Autodesk Inventor part; units mm, degrees
ref_plane "YZ Plane" through (0, 0, 0) normal (1, 0, 0) x (0, 1, 0)
ref_plane "XZ Plane" through (0, 0, 0) normal (0, 1, 0) x (-1, 0, 0)
ref_plane "XY Plane" through (0, 0, 0) normal (0, 0, 1) x (1, 0, 0)
sketch "Boceto1" plane through (0, 0, 0) normal (0, 0, 1) x (1, 0, 0)
  arc A0 (-116.1173, 21.3488) -> (-117.6673, 19.7988) centre (-116.1173, 19.7988) ccw
  arc A1 (-117.6673, 19.7988) -> (-116.1173, 18.2488) centre (-116.1173, 19.7988) ccw
  arc A2 (-116.1173, 18.2488) -> (-114.5673, 19.7988) centre (-116.1173, 19.7988) ccw
  arc A3 (-114.5673, 19.7988) -> (-116.1173, 21.3488) centre (-116.1173, 19.7988) ccw
  arc A4 (-67.1173, 21.3488) -> (-68.6673, 19.7988) centre (-67.1173, 19.7988) ccw
  arc A5 (-68.6673, 19.7988) -> (-67.1173, 18.2488) centre (-67.1173, 19.7988) ccw
  arc A6 (-67.1173, 18.2488) -> (-65.5673, 19.7988) centre (-67.1173, 19.7988) ccw
  arc A7 (-65.5673, 19.7988) -> (-67.1173, 21.3488) centre (-67.1173, 19.7988) ccw
  arc A8 (-18.1173, 21.3488) -> (-19.6673, 19.7988) centre (-18.1173, 19.7988) ccw
  arc A9 (-19.6673, 19.7988) -> (-18.1173, 18.2488) centre (-18.1173, 19.7988) ccw
  arc A10 (-18.1173, 18.2488) -> (-16.5673, 19.7988) centre (-18.1173, 19.7988) ccw
  arc A11 (-16.5673, 19.7988) -> (-18.1173, 21.3488) centre (-18.1173, 19.7988) ccw
  arc A12 (-18.1173, -7.6512) -> (-19.6673, -9.2012) centre (-18.1173, -9.2012) ccw
  arc A13 (-19.6673, -9.2012) -> (-18.1173, -10.7512) centre (-18.1173, -9.2012) ccw
  arc A14 (-18.1173, -10.7512) -> (-16.5673, -9.2012) centre (-18.1173, -9.2012) ccw
  arc A15 (-16.5673, -9.2012) -> (-18.1173, -7.6512) centre (-18.1173, -9.2012) ccw
  arc A16 (-116.1173, -7.6512) -> (-117.6673, -9.2012) centre (-116.1173, -9.2012) ccw
  arc A17 (-117.6673, -9.2012) -> (-116.1173, -10.7512) centre (-116.1173, -9.2012) ccw
  arc A18 (-116.1173, -10.7512) -> (-114.5673, -9.2012) centre (-116.1173, -9.2012) ccw
  arc A19 (-114.5673, -9.2012) -> (-116.1173, -7.6512) centre (-116.1173, -9.2012) ccw
  arc A20 (-116.1173, -36.6512) -> (-117.6673, -38.2012) centre (-116.1173, -38.2012) ccw
  arc A21 (-117.6673, -38.2012) -> (-116.1173, -39.7512) centre (-116.1173, -38.2012) ccw
  arc A22 (-116.1173, -39.7512) -> (-114.5673, -38.2012) centre (-116.1173, -38.2012) ccw
  arc A23 (-114.5673, -38.2012) -> (-116.1173, -36.6512) centre (-116.1173, -38.2012) ccw
  arc A24 (-18.1173, -36.6512) -> (-19.6673, -38.2012) centre (-18.1173, -38.2012) ccw
  arc A25 (-19.6673, -38.2012) -> (-18.1173, -39.7512) centre (-18.1173, -38.2012) ccw
  arc A26 (-18.1173, -39.7512) -> (-16.5673, -38.2012) centre (-18.1173, -38.2012) ccw
  arc A27 (-16.5673, -38.2012) -> (-18.1173, -36.6512) centre (-18.1173, -38.2012) ccw
  arc A28 (-102.1173, 31.8488) -> (-103.6673, 30.2988) centre (-102.1173, 30.2988) ccw
  arc A29 (-103.6673, 30.2988) -> (-102.1173, 28.7488) centre (-102.1173, 30.2988) ccw
  arc A30 (-102.1173, 28.7488) -> (-100.5673, 30.2988) centre (-102.1173, 30.2988) ccw
  arc A31 (-100.5673, 30.2988) -> (-102.1173, 31.8488) centre (-102.1173, 30.2988) ccw
  arc A32 (-32.1173, 31.8488) -> (-33.6673, 30.2988) centre (-32.1173, 30.2988) ccw
  arc A33 (-33.6673, 30.2988) -> (-32.1173, 28.7488) centre (-32.1173, 30.2988) ccw
  arc A34 (-32.1173, 28.7488) -> (-30.5673, 30.2988) centre (-32.1173, 30.2988) ccw
  arc A35 (-30.5673, 30.2988) -> (-32.1173, 31.8488) centre (-32.1173, 30.2988) ccw
  line L0 (-22.3173, 1.3488) -> (-22.3173, 13.2488)
  line L1 (-22.3173, 13.2488) -> (-50.9173, 13.2488)
  line L2 (-50.9173, 13.2488) -> (-50.9173, 1.3488)
  line L3 (-50.9173, 1.3488) -> (-22.3173, 1.3488)
  line L4 (-83.3173, 1.3488) -> (-83.3173, 13.2488)
  line L5 (-83.3173, 13.2488) -> (-111.9173, 13.2488)
  line L6 (-111.9173, 13.2488) -> (-111.9173, 1.3488)
  line L7 (-111.9173, 1.3488) -> (-83.3173, 1.3488)
  line L8 (-86.2223, 27.9117) -> (-86.2223, 32.6859)
  line L9 (-86.2223, 32.6859) -> (-92.0123, 32.6859)
  line L10 (-92.0123, 32.6859) -> (-92.0123, 27.9117)
  line L11 (-92.0123, 27.9117) -> (-86.2223, 27.9117)
  line L12 (-112.1673, 27.8663) -> (-112.1673, 32.7313)
  line L13 (-112.1673, 32.7313) -> (-118.0673, 32.7313)
  line L14 (-118.0673, 32.7313) -> (-118.0673, 27.8663)
  line L15 (-118.0673, 27.8663) -> (-112.1673, 27.8663)
  line L16 (-42.1673, 27.8663) -> (-42.1673, 32.7313)
  line L17 (-42.1673, 32.7313) -> (-48.0673, 32.7313)
  line L18 (-48.0673, 32.7313) -> (-48.0673, 27.8663)
  line L19 (-48.0673, 27.8663) -> (-42.1673, 27.8663)
  line L20 (-16.1673, 27.8663) -> (-16.1673, 32.7313)
  line L21 (-16.1673, 32.7313) -> (-22.0673, 32.7313)
  line L22 (-22.0673, 32.7313) -> (-22.0673, 27.8663)
  line L23 (-22.0673, 27.8663) -> (-16.1673, 27.8663)
  line L24 (-36.0566, -42.9012) -> (-36.0566, -3.3934)
  line L25 (-36.0566, -3.3934) -> (-41.3173, -3.3934)
  line L26 (-41.3173, -3.3934) -> (-80.1673, -3.3934)
  line L27 (-80.1673, -3.3934) -> (-91.1173, -3.3934)
  line L28 (-91.1173, -3.3934) -> (-91.1173, -42.9012)
  line L29 (-91.1173, -42.9012) -> (-122.3173, -42.9012)
  line L30 (-122.3173, -42.9012) -> (-122.3173, 35.4988)
  line L31 (-122.3173, 35.4988) -> (-81.9173, 35.4988)
  line L32 (-81.9173, 35.4988) -> (-81.9173, 27.4988)
  line L33 (-81.9173, 27.4988) -> (-52.3173, 27.4988)
  line L34 (-52.3173, 27.4988) -> (-52.3173, 35.4988)
  line L35 (-52.3173, 35.4988) -> (-11.9173, 35.4988)
  line L36 (-11.9173, 35.4988) -> (-11.9173, -42.9012)
  line L37 (-11.9173, -42.9012) -> (-36.0566, -42.9012)
  point P0 (0, 0)
extrude "Extrusión1" add sketch "Boceto1" along normal blind 5
properties part number "carro x lado motor pieza 1"
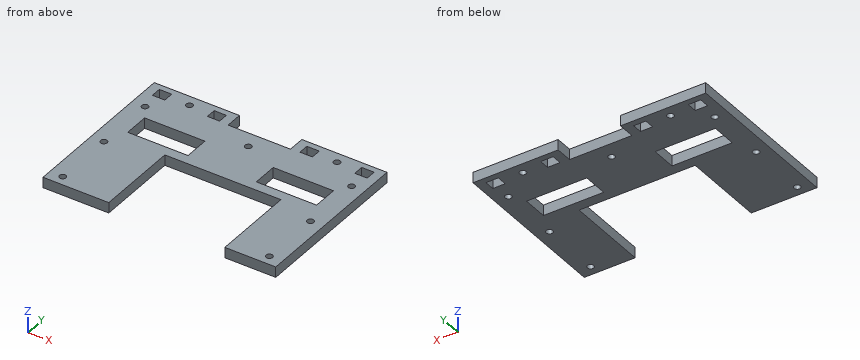
Model file for the job. Use its own axes, mm. Round coordinates to 2 decimals unless told otherwise and drop trailing zeros. Loops run counter-clockwise (first coordinate to the right, second up) from the corner with the lowest first, then second, coordinate; pieces in that order, holes last.
1. Drop a flat-ended pin along its axis: P1, Ø1, axis at x = -52.5, z = 3, coming from the -Y side. Give the stop position or say it passes through.
Check values:
P1: stops at y = -3.39
2. Band-saw the part on B-B, the plane y = -32.5. List the corners of the cut face in (x, z), and give its area (3 significant figures).
Check values:
outline: (-122.32, 0) - (-91.12, 0) - (-91.12, 5) - (-122.32, 5) - close; (-36.06, 0) - (-11.92, 0) - (-11.92, 5) - (-36.06, 5) - close
area: 277 mm2
3. Band-saw the part on A-A, the plane x = -27. List the corners of the cut face in (y, z), and give its area (4 significant figures).
Check values:
outline: (-42.9, 0) - (1.35, 0) - (1.35, 5) - (-42.9, 5) - close; (13.25, 0) - (35.5, 0) - (35.5, 5) - (13.25, 5) - close
area: 332.5 mm2
4. Band-saw the part on D-D, the plane z = 1. Count the separate pieces of the cut face and the enclosed holes in it, and give its area (3 significant figures).
Check values:
separate pieces: 1
enclosed holes: 15
area: 5,380 mm2
5. Wall check: probe 1 along Y at (x, z) = (-116, 0.2); probe 2 along Y at (x, z) = (-45, 1.3); probe 3 along X at (y, z) = (10, 4.05). Give the ranges that are in metal, low to high.
Check values:
probe 1: y = -42.9 to -39.75, -36.66 to -10.75, -7.66 to 18.25, 21.34 to 27.87, 32.73 to 35.5
probe 2: y = -3.39 to 1.35, 13.25 to 27.87, 32.73 to 35.5
probe 3: x = -122.32 to -111.92, -83.32 to -50.92, -22.32 to -11.92
6. Band-saw the part on C-C, the plane x = -88.5. List the corners of the cut face in (y, z).
Check values:
outline: (-3.39, 0) - (1.35, 0) - (1.35, 5) - (-3.39, 5) - close; (13.25, 0) - (27.91, 0) - (27.91, 5) - (13.25, 5) - close; (32.69, 0) - (35.5, 0) - (35.5, 5) - (32.69, 5) - close
